Design review of the part built by this model. Coordinates are the model's own, in mm. A direction names the side the tool comes from. Round coordinates to 2 decimals unless told otherwise and drop trailing zeros. Order: outer loops, then holes, each group sorted by start corner. A loop starts at its lowest first (then second) coordinate and runs counter-clockwise, first axis right, second up. Notation, with made-up numbers: (68.25, 18.5) - (87.25, 18.5) arc R18 cw to (87.25, 51.5) - close; hole circle Ø6 at (56, 83). An arc over 180 degrees is marked (long way). Write item = value, one per line.
Solid Edge part; units mm, degrees
sketch "Sketch1" plane through (0, 0, 0) normal (1, 0, 0) x (0, 1, 0)
  circle A0 centre (0, 0) radius 30
  circle A1 centre (0, 0) radius 15
extrude "Protrusion1" add sketch "Sketch1" along normal mid plane 80
sketch "Sketch2" plane through (0, 0, 66) normal (0, 0, 1) x (1, 0, 0)
  circle A0 centre (0, 40) radius 30
sketch "Sketch3" plane through (0, 0, 106) normal (0, 0, 1) x (1, 0, 0)
  circle A0 centre (0, 40) radius 20
loft "LoftedProtrusion1" add profiles "Sketch2", "Sketch3"
sketch "Sketch4" plane through (0, 0, 66) normal (0, 0, 1) x (1, 0, 0)
  line L0 (30, 0) -> (30, 40)
  arc A0 (-30, 40) -> (30, 40) centre (0, 40) cw
  line L1 (-30, 0) -> (-30, 40)
  line L2 (30, 0) -> (-30, 0)
extrude "ExtrudedProtrusion_2" add sketch "Sketch4" against normal blind 20
sketch "Sketch5" plane through (0, 0, 106) normal (0, 0, 1) x (1, 0, 0)
  circle A0 centre (0, 40) radius 10
extrude "Cutout1" cut sketch "Sketch5" against normal up to vertex (60 mm away)
sketch "Sketch6" plane through (30, 20, 56) normal (1, 0, 0) x (0, 1, 0)
  line L0 (-20, -10) -> (-20, -26)
  arc A0 (-20, -26) -> (0, -33.6393) centre (-20, -56) cw
  line L1 (0, -10) -> (0, -33.6393)
  line L2 (-20, -10) -> (0, -10)
extrude "ExtrudedProtrusion_3" add sketch "Sketch6" against normal blind 60
sketch "Sketch7" plane through (0, 0, 0) normal (1, 0, 0) x (0, 1, 0)
  line L0 (0, 66) -> (-26.7217, 13.6364)
  arc A0 (-26.7217, 13.6364) -> (0, 30) centre (0, 0) cw
  line L1 (0, 66) -> (0, 30)
extrude "ExtrudedProtrusion_4" add sketch "Sketch7" along normal mid plane 12
1) Clearance check with flat-ended pins moving along their axes: pin 1 Ø10 at (x, z) = (23, 25) entering from +Y; pin 2 Ø12 at (x, z) = (-17, 1.5) entering from +Y; pin 3 Ø10 at (x, z) = (11, -11) entering from +Y. State where each tip first meets the part, or that it passes through.
Findings:
pin_1 = 22.36
pin_2 = 30
pin_3 = 29.39
2) We need section A-A on z = 0. Write out the cut boundary in (x, y).
Findings:
outline = (-40, -30) - (40, -30) - (40, -15) - (-40, -15) - close; (-40, 15) - (40, 15) - (40, 30) - (-40, 30) - close
3) We need section D-D on z = 58.5. Write out the cut boundary in (x, y), and give its area (3 significant figures).
Findings:
outline = (-30, 0) - (-6, 0) - (-6, -3.83) - (6, -3.83) - (6, 0) - (30, 0) - (30, 40) arc R30 ccw to (-30, 40) - close; hole circle Ø20 at (0, 40)
area = 3,550 mm^2
4) To check wall thickness, follow L1, parallel to Z at x = -4.5, y = 0; L2, parallel to Z at x = 34.5, y = 1; L3, parallel to Y at x = -1, z = 86.5. State the ranges of each line that lie inside material, in increasing order. Write a range as from..to.
Findings:
L1 = -30..-15, 15..66
L2 = -29.98..-14.97, 14.97..29.98
L3 = 15.15..30.05, 49.95..64.85
5) We need section C-C on x = 34.5. Write out the cut boundary in (y, z), and give its area (3 significant figures).
Findings:
outline = circle Ø60 at (0, 0); hole circle Ø30 at (0, 0)
area = 2,120 mm^2
6) The part is to be moulded in two halves that separate along Y. For faces 5 (the cylindrical face through (-0.56, -14.985, -0.66)), 6 (the cylindrical face through (0.66, 69.993, 56.14)), 7 (the flat face through (40, -14, 6)), 8 (the flat face through (-0.084, -13.174, 40.185)), say which applies: released by +Y, released by -Y, zero draft, split by the parting line, or undercut.
Findings:
face_5 = undercut
face_6 = released by +Y
face_7 = zero draft
face_8 = released by -Y
7) For faces 1 (the flat face through (0, 51, 46)), 2 (the cylindrical face through (-0.56, -3.905, -29.745)), 3 (the flat face through (-18, 0, 48)), 4 (the flat face through (18, 0, 48)), list the 3-axis set-ups (+Z, -Z, +X, -X, +Y, -Y) from which the entire face can be reached by the end or side of a thin tool; tool diameter is ignored.
Findings:
face_1 = +X, -X, +Y
face_2 = none
face_3 = +Z, -X, -Y
face_4 = +Z, +X, -Y
8) We need section B-B on y = -9. Write out the cut boundary in (x, z).
Findings:
outline = (-40, -28.62) - (40, -28.62) - (40, -12) - (-40, -12) - close; (-40, 12) - (40, 12) - (40, 28.62) - (6, 28.62) - (6, 48.36) - (-6, 48.36) - (-6, 28.62) - (-40, 28.62) - close
